Geometry check sheet. Reference: the model listing, model coordinates, mm. Face numbers are marked on the shaded views. Give positions to 0.01 mm unless a question says otherwise; leave off trailing zeros. Loops run counter-clockwise (first coordinate to the right, second up) from the corner with the lowest first, then second, coordinate; pieces in that order, holes last. Notation, with made-up numbers: (39, 63) -> (64, 63) arc R28 cw to (64, 102) -> close; hole circle Ø11 at (13, 67). An arc over 180 degrees is marked (long way). One line per item, written item: value. Start each with the question number.
(1) Draft check along Z on the marked faces 1 and 2. Enter one of: pulls with the +Z half, pulls with the -Z half, needs draft (parallel to the pull), parting line crosses it, or undercut.
(2) Scan lines: line 1 along Y through (x, z) = (0, -18.55) (3 decimals); line 2 along X through (y, z) = (122.5, 1); line 3 along Z through (x, y) = (0, 70). Record each from-to range of solid material in increasing order. Write a range as from..to.
(3) Sectioned sample at A-A, the plane z = 0. Record the cut outline in (x, y), then the cut area to 3 significant figures.
(4) Sectioned sample at C-C, the plane y = 189.5. Record the cut outline in (x, z).
(5) Sectioned sample at B-B, the plane x = 8. Record the cut outline in (y, z), then the cut area to 3 significant figures.
(6) Gauge pin test, flat ends, axial feed: pin 1 Ø1.5 at (x, y) = (15, 206.5) entering from -Z; pin 2 Ø4 at (y, z) = (61, -11.5) entering from -X; pin 3 Ø5 at (x, y) = (5, 202) entering from -Z; pin 4 Ø2.5 at (x, y) = (0, 3.92) entering from -Z. Record the tip position at first contact, or that the pin passes through.
from build123d import *

# Parameters (mm, degrees)
SKETCH2_R           = 19.25
SKETCH2_R_2         = 18
BOSS_EXTRUDE1_DEPTH = 231.82
SKETCH3_R           = 0.815
CUT_EXTRUDE2_DEPTH  = 231.82
CIRPATTERN3_COUNT   = 6
SKETCH4_R           = 0.815
CUT_EXTRUDE3_DEPTH  = 231.82
CIRPATTERN4_COUNT   = 6


with BuildPart() as part:
    # Sketch2 → Boss-Extrude1 (new body)
    with BuildSketch(Plane(origin=(0, 0, 0), x_dir=(1, 0, 0), z_dir=(0, 1, 0))):
        Circle(SKETCH2_R)
        Circle(SKETCH2_R_2, mode=Mode.SUBTRACT)
    extrude(amount=BOSS_EXTRUDE1_DEPTH)

    # Sketch3 → Cut-Extrude2 (cut)
    with BuildSketch(Plane.XY):
        with Locations((0, 3.92)):
            Circle(SKETCH3_R)
    cut_extrude2 = extrude(amount=-CUT_EXTRUDE2_DEPTH, mode=Mode.SUBTRACT)

    # CirPattern3: Cut-Extrude2 ×6 about axis
    cirpattern3_axis = Axis((0, 231.82, 0), (0, -1, 0))
    for i in range(1, CIRPATTERN3_COUNT):
        add(cut_extrude2.rotate(cirpattern3_axis, i * 360 / CIRPATTERN3_COUNT), mode=Mode.SUBTRACT)

    # Sketch4 → Cut-Extrude3 (cut)
    with BuildSketch(Plane.XY):
        with Locations((0, 228.73)):
            Circle(SKETCH4_R)
    cut_extrude3 = extrude(amount=CUT_EXTRUDE3_DEPTH, mode=Mode.SUBTRACT)

    # CirPattern4: Cut-Extrude3 ×6 about axis
    cirpattern4_axis = Axis((0, 231.82, 0), (0, -1, 0))
    for i in range(1, CIRPATTERN4_COUNT):
        add(cut_extrude3.rotate(cirpattern4_axis, i * 360 / CIRPATTERN4_COUNT), mode=Mode.SUBTRACT)


solid = part.part
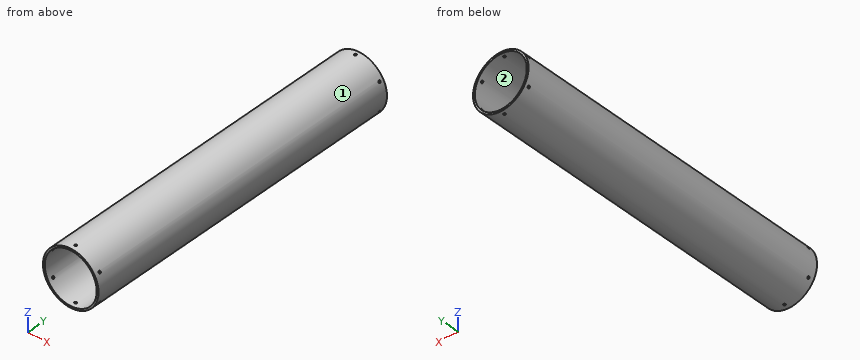
Calculated:
1. face 1: parting line crosses it
1. face 2: undercut
2. line 1: y = 0..3.105, 4.735..227.915, 229.545..231.82
2. line 2: x = -19.22..-17.97, 17.97..19.22
2. line 3: z = -19.25..-18, 18..19.25
3. outline: (-19.25, 0) -> (-18, 0) -> (-18, 231.82) -> (-19.25, 231.82) -> close; (18, 0) -> (19.25, 0) -> (19.25, 231.82) -> (18, 231.82) -> close
3. area: 580 mm2
4. outline: circle Ø38.5 at (0, 0); hole circle Ø36 at (0, 0)
5. outline: (0, -17.51) -> (231.82, -17.51) -> (231.82, -16.12) -> (0, -16.12) -> close; (0, 16.12) -> (231.82, 16.12) -> (231.82, 17.51) -> (0, 17.51) -> close
5. area: 642 mm2
6. pin 1: stops at z = -12.94
6. pin 2: stops at x = -16.74
6. pin 3: stops at z = -19.09
6. pin 4: stops at z = -19.25
